```python
from build123d import *

# Parameters (mm, degrees)
SKETCH_1_R          = 8.75
EXTRUDE_1_DEPTH     = 4
EXTRUDE_START       = -2.5
SKETCH_3_R          = 8.75
SKETCH_3_R_2        = 4.5
EXTRUDE_2_DEPTH     = 2.5
CUT_EXTRUDE_2_DEPTH = 221.943431674
SKETCH_4_R          = 1.7
CUT_EXTRUDE_3_DEPTH = 221.943431674
SKETCH_5_R          = 3
CUT_EXTRUDE_4_DEPTH = 2


with BuildPart() as part:
    # 草图1 → 凸台-拉伸1 (new body)
    with BuildSketch(Plane.XY):
        with BuildLine():
            Line((-20, 0), (-20, -200))
            ThreePointArc((-20, -200), (0, -220), (20, -200))
            Line((20, -200), (20, 0))
            ThreePointArc((20, 0), (0, 20), (-20, 0))
        make_face()
        Circle(SKETCH_1_R, mode=Mode.SUBTRACT)
        with Locations((0, -200)):
            Circle(SKETCH_1_R, mode=Mode.SUBTRACT)
    extrude(amount=EXTRUDE_1_DEPTH)

    # 草图3 → 凸台-拉伸2 (add)
    # profile 1 of 2: a face of its own
    with BuildSketch(Plane.XY.offset(4).offset(EXTRUDE_START)):
        Circle(SKETCH_3_R)
        Circle(SKETCH_3_R_2, mode=Mode.SUBTRACT)
    # profile 2 of 2: a face of its own
    with BuildSketch(Plane.XY.offset(4).offset(EXTRUDE_START)):
        with Locations((0, -200)):
            Circle(SKETCH_3_R)
        with Locations((0, -200)):
            Circle(SKETCH_3_R_2, mode=Mode.SUBTRACT)
    extrude(amount=EXTRUDE_2_DEPTH)

    # 草图2 → 切除-拉伸2 (cut, through all)
    with BuildSketch(Plane.XY.offset(4)):
        with BuildLine():
            Line((-5, -31.845004689), (-5, -159.845004689))
            ThreePointArc((-5, -159.845004689), (0, -164.845004689), (5, -159.845004689))
            Line((5, -159.845004689), (5, -31.845004689))
            ThreePointArc((5, -31.845004689), (0, -26.845004689), (-5, -31.845004689))
        make_face()
    extrude(amount=-CUT_EXTRUDE_2_DEPTH, mode=Mode.SUBTRACT)

    # 草图4 → 切除-拉伸3 (cut, through all)
    with BuildSketch(Plane(origin=(0, 0, 0), x_dir=(-1, 0, 0), z_dir=(0, 0, -1))):
        with Locations((0, -214)):
            Circle(SKETCH_4_R)
        with Locations((-12.124355653, -193)):
            Circle(SKETCH_4_R)
        with Locations((12.124355653, -193)):
            Circle(SKETCH_4_R)
    extrude(amount=-CUT_EXTRUDE_3_DEPTH, mode=Mode.SUBTRACT)

    # 草图5 → 切除-拉伸4 (cut)
    with BuildSketch(Plane(origin=(0, 0, 0), x_dir=(-1, 0, 0), z_dir=(0, 0, -1))):
        with Locations((-12.124355653, -193)):
            Circle(SKETCH_5_R)
        with Locations((12.124355653, -193)):
            Circle(SKETCH_5_R)
        with Locations((0, -214)):
            Circle(SKETCH_5_R)
    extrude(amount=-CUT_EXTRUDE_4_DEPTH, mode=Mode.SUBTRACT)


solid = part.part
```
Can you work these out from the model? Positions are in its coordinate system, mm. A direction names the side the tool comes from. Give positions to 0.01 mm unless a question says otherwise; leave off trailing zeros. Write each loop counter-clockwise with the first axis right and the second up, starting at its lowest first coordinate (ties: lowest second). Pieces come first, ordered by that corner, then holes. Notation, with made-up numbers: (82, -23.5) -> (128, -23.5) arc R6 cw to (128, -18.5) -> close; hole circle Ø1 at (-24, 10.25). An arc over 180 degrees is marked (long way). Write item = value, one per line.
(1) I'm going to push flat-ended pins straight in: P1, Ø9, axis at x = 3.5, y = 0, coming from the -Z side; P2, Ø5, axis at x = 0, y = -214, coming from the -Z side. Where does each tip first touch, or does it pass through?
Worked out:
P1 = 1.5
P2 = 2
(2) I need wall thicknesses on probe 1 along Y at (x, z) = (0, 3.2) (3 decimals); probe 2 along X at (y, z) = (-110, 3.2); probe 3 along Y at (x, z) = (0, 0.9) (3 decimals). Which ranges of each line are inside material? Lowest first, please. Write a range as from..to.
Worked out:
probe_1 = -220..-215.7, -212.3..-204.5, -195.5..-164.845, -26.845..-4.5, 4.5..20
probe_2 = -20..-5, 5..20
probe_3 = -220..-217, -211..-208.75, -191.25..-164.845, -26.845..-8.75, 8.75..20
(3) For faces 1 (the face through (0, 20, 2)), 2 (the face through (0.11, -26.846, 2.028)), 3 (the face through (12.515, -190.026, 0.986)), which set-ups out of +Z, -Z, +X, -X, +Y, -Y let a thin tool reach every point of the face, with its end or its side?
Worked out:
face_1 = +Z, -Z, +Y
face_2 = +Z, -Z
face_3 = -Z
(4) Thinking about a two-plate mould opening in X: for faces 4 (the face through (-2, -214, 2)), 5 (the face through (9, -98, 0)), 6 (the face through (-20, -99, 2)), which applies, released by +X, released by -X, zero draft, split by the parting line, or undercut?
Worked out:
face_4 = undercut
face_5 = zero draft
face_6 = released by -X
(5) Suppose I cut it at B-B on y = -95.5. Write out the boundary of the cut face in (x, z).
Worked out:
outline = (-20, 0) -> (-5, 0) -> (-5, 4) -> (-20, 4) -> close; (5, 0) -> (20, 0) -> (20, 4) -> (5, 4) -> close
(6) Suppose I cut it at A-A on z = 2.75. Write out the boundary of the cut face in (x, y) (3 decimals), then the cut area to 3 significant figures.
Worked out:
outline = (-20, -200) arc R20 ccw to (20, -200) -> (20, 0) arc R20 ccw to (-20, 0) -> close; hole circle Ø3.4 at (-12.124, -193); hole (-5, -159.845) arc R5 ccw to (5, -159.845) -> (5, -31.845) arc R5 ccw to (-5, -31.845) -> close; hole circle Ø9 at (0, -200); hole circle Ø9 at (0, 0); hole circle Ø3.4 at (0, -214); hole circle Ø3.4 at (12.124, -193)
area = 7,740 mm^2
